Verification items for the finished model (mm, model axes). A direction names the side the tool comes from. Round coordinates to 2 decimals unless told otherwise and drop trailing zeros. Write each loop counter-clockwise with the first axis right and the second up, starting at its lowest first coordinate (ties: lowest second). Pieces come first, ordered by that corner, then holes. Notation, with made-up numbers: M 23.5,-2.5 L 41.5,-2.5 A11 ccw 41.5,1.5 Z; hole C 86,25.5 d2. An arc over 180 degrees is marked long. One line per question, with ' | ' between items. Start each with the question number.
Q1. Thickness scan on line 1 along Y through (x, z) = (0, -1); line 2 along X through (y, z) = (91, -1.25); line 3 along X through (y, z) = (30, 2.7). Record the ranges inside material, lowest first. Write a range as from..to.
Q2. Gauge pin test, flat end, axial feed: pin 1 (4.5 mm diameter, centred on x = 0, y = 10, fed in from -Z). Record the tip position at first contact, or that the pin passes through.
Q3. Cross-section at A-A (y = 70). Record the boundary of the cut face in (x, z).
Q4. Cross-section at B-B (z = -2.25). Record the boundary of the cut face in (x, y).
Q5. Release check for a two-part mould opening along Y. For faces 1 (the face through (1, 68, 0.5)), 2 (the face through (-2, 49, 3.25)) record: released by +Y, released by -Y, zero draft, split by the parting line, or undercut.
Q6. Tool access check on faces 3 (the face through (-0.07, 48.3, 1.89)), 4 (the face through (1.3, 53.14, -1.35)). Record the directions out of +Z, -Z, +X, -X, +Y, -Y that give a thin tool (end or side, any length) a straight path to the whole face; none if there is none.
Autodesk Inventor part; units mm, degrees
ref_plane "YZ Plane" through (0, 0, 0) normal (1, 0, 0) x (0, 1, 0)
ref_plane "XZ Plane" through (0, 0, 0) normal (0, 1, 0) x (-1, 0, 0)
ref_plane "XY Plane" through (0, 0, 0) normal (0, 0, 1) x (1, 0, 0)
sketch "Sketch1" plane through (0, 0, 0) normal (0, 1, 0) x (-1, 0, 0)
  line L0 (-4.5, -3.25) -> (4.5, -3.25)
  line L1 (4.5, -3.25) -> (4.5, 3.25)
  line L2 (4.5, 3.25) -> (-4.5, 3.25)
  line L3 (-4.5, 3.25) -> (-4.5, -3.25)
  line L4 (-4.5, -3.25) -> (4.5, 3.25) construction
  line L5 (4.5, -3.25) -> (-4.5, 3.25) construction
  point P0 (0, 0)
  dimension "d0" = 9
  dimension "d1" = 6.5
extrude "Extrusion1" add sketch "Sketch1" along normal blind 100
sketch "Sketch2" plane through (4.5, 0, -3.25) normal (0, 0, -1) x (-1, 0, 0)
  line L0 (0, 0) -> (9, 0) construction
  line L1 (9, 0) -> (9, 100) construction
  line L2 (0, 100) -> (9, 100) construction
  line L3 (0, 0) -> (0, 100) construction
  line L4 (9, 100) -> (0, 100)
  line L5 (4.5, 100) -> (4.5, 0) construction
  point P0 (4.5, 90)
  point P1 (4.5, 70)
  point P2 (4.5, 50)
  point P3 (4.5, 30)
  point P4 (4.5, 10)
  dimension "d4" = 20
  dimension "d5" = 20
  dimension "d6" = 20
  dimension "d7" = 20
  dimension "d9" = 10
  dimension "d10" = 10
hole "Hole1" at (0, 90, -3.25) at (0, 70, -3.25) at (0, 50, -3.25) at (0, 30, -3.25) at (0, 10, -3.25) direction (0, 0, 1) diameter 3.4 depth 8 counterbore diameter 6.8 counterbore depth 3.75
properties part number "LinearRail" material "Steel, Carbon"
Determined:
1) line 1: y = 0..6.6, 13.4..26.6, 33.4..46.6, 53.4..66.6, 73.4..86.6, 93.4..100 | line 2: x = -4.5..-3.25, 3.25..4.5 | line 3: x = -4.5..-1.7, 1.7..4.5
2) pin 1: stops at z = 0.5
3) outline: M -4.5,-3.25 L -3.4,-3.25 L -3.4,0.5 L -1.7,0.5 L -1.7,3.25 L -4.5,3.25 Z; M 1.7,0.5 L 3.4,0.5 L 3.4,-3.25 L 4.5,-3.25 L 4.5,3.25 L 1.7,3.25 Z
4) outline: M -4.5,0 L 4.5,0 L 4.5,100 L -4.5,100 Z; hole C 0,10 d6.8; hole C 0,30 d6.8; hole C 0,50 d6.8; hole C 0,70 d6.8; hole C 0,90 d6.8
5) face 1: undercut | face 2: zero draft
6) face 3: +Z, -Z | face 4: -Z
